Check sheet for the drawn part. Datum: minimum x, y, z corner. Units: mm. Round coordinates to 2 decimals unless told otherwise and drop trailing zeros. Order: outer loops, then holes, each group sorted by start corner. A loop starts at its lowest first (then second) coordinate and runs counter-clockwise, first axis right, second up. Notation, with made-up numbers: (39.5, 38) -> (88.5, 38) arc R31 ccw to (88.5, 74) -> close; hole circle Ø3 at (0.5, 17). An arc over 180 degrees is marked (long way). Answer as CSV lines item,"result". Start each with the question number.
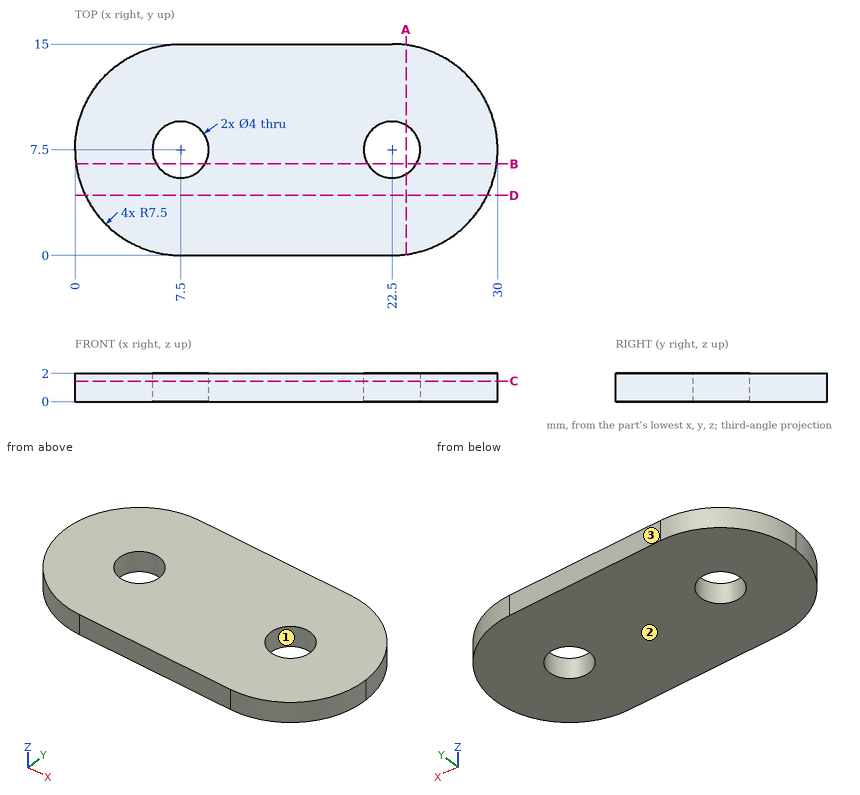
1) Mould release check, pull along Y, two halves, no side actions. Record for the marked faces 1, 2 and 3: released by +Y, released by -Y, zero draft, split by the parting line, or undercut.
2) Depth check by flat-ended pin: pin 1 Ø1 at (x, z) = (5.5, 0.5) entering from -Y. Enter the tip coordinate at first touch or a pass-through.
3) Section check C-C on z = 1.45. Count the separate pieces of the cut face and the enclosed holes in it, then the cut area to 3 significant figures.
4) Section check B-B on y = 6.5. Record the cut outline in (x, z).
5) Section check A-A on x = 23.5. Record the cut outline in (y, z), then the cut area to 3 significant figures.
6) Material ranges on line 1 along Y through (x, z) = (22.5, 1.5); line 2 along X through (y, z) = (6, 1.1); line 3 along X through (y, z) = (3, 0.8), recorded low to high.
7) Section check D-D on y = 4.25. Record the cut outline in (x, z), then the cut area to 3 significant figures.
Solutions:
1,face 1,"undercut"
1,face 2,"zero draft"
1,face 3,"released by +Y"
2,pin 1,"stops at y = 0.15"
3,separate pieces,"1"
3,enclosed holes,"2"
3,area,"377 mm^2"
4,outline,"(0.07, 0) -> (5.77, 0) -> (5.77, 2) -> (0.07, 2) -> close; (9.23, 0) -> (20.77, 0) -> (20.77, 2) -> (9.23, 2) -> close; (24.23, 0) -> (29.93, 0) -> (29.93, 2) -> (24.23, 2) -> close"
5,outline,"(0.07, 0) -> (5.77, 0) -> (5.77, 2) -> (0.07, 2) -> close; (9.23, 0) -> (14.93, 0) -> (14.93, 2) -> (9.23, 2) -> close"
5,area,"22.8 mm^2"
6,line 1,"y = 0 to 5.5, 9.5 to 15"
6,line 2,"x = 0.15 to 6.18, 8.82 to 21.18, 23.82 to 29.85"
6,line 3,"x = 1.5 to 28.5"
7,outline,"(0.74, 0) -> (29.26, 0) -> (29.26, 2) -> (0.74, 2) -> close"
7,area,"57.0 mm^2"
